```python
from build123d import *
from OCP.BRepFilletAPI import BRepFilletAPI_MakeChamfer

# Parameters (mm, degrees)
SKETCH3_W           = 20
SKETCH3_H           = 20
BOSS_EXTRUDE1_DEPTH = 2
SKETCH4_W           = 20
SKETCH4_H           = 20
SKETCH4_W_2         = 17.8
SKETCH4_H_2         = 17.8
BOSS_EXTRUDE2_DEPTH = 0.8
CHAMFER1_SIZE       = 2
BOSS_EXTRUDE3_DEPTH = 4.8
FILLET2_R           = 1
FILLET4_R           = 1
BOSS_EXTRUDE4_DEPTH = 6.1
CHAMFER2_SIZE       = 1.5
CHAMFER2_SIZE2      = 0.415986816
FILLET5_R           = 0.25
FILLET6_R           = 0.25


with BuildPart() as part:
    # Sketch3 → Boss-Extrude1 (new body)
    with BuildSketch(Plane.XY):
        Rectangle(SKETCH3_W, SKETCH3_H)
    extrude(amount=BOSS_EXTRUDE1_DEPTH)

    # Sketch4 → Boss-Extrude2 (add)
    with BuildSketch(Plane.XY.offset(2)):
        Rectangle(SKETCH4_W, SKETCH4_H)
        Rectangle(SKETCH4_W_2, SKETCH4_H_2, mode=Mode.SUBTRACT)
    extrude(amount=BOSS_EXTRUDE2_DEPTH)

    # Chamfer1
    chamfer1_edges = [part.edges().sort_by_distance(p)[0] for p in [
        (0, 10, 0),
        (10, 0, 0),
        (0, -10, 0),
        (-10, 0, 0),
    ]]
    chamfer(chamfer1_edges, length=CHAMFER1_SIZE)

    # Sketch7 → Boss-Extrude3 (add)
    with BuildSketch(Plane.XY.offset(2)):
        Polygon((-7.6, 5.05), (-7.6, -5.05), (-5.73, -5.05), (-3.861210285, -2.885), (-3.861210285, 2.885), (-5.73, 5.05), align=None)
        Polygon((-5.181210285, -2.394094045), (-5.181210285, 2.394094045), (-6.28, 3.667046113), (-6.28, -3.667046113), align=None, mode=Mode.SUBTRACT)
    boss_extrude3 = extrude(amount=BOSS_EXTRUDE3_DEPTH)

    # Mirror1: Boss-Extrude3 across plane
    add(boss_extrude3.mirror(Plane(origin=(0, 0, 0), x_dir=(0, 0, 1), z_dir=(1, 0, 0))))

    # Fillet2
    fillet2_edges = [part.edges().sort_by_distance(p)[0] for p in [
        (-6.665, 5.05, 6.8),
        (-7.6, 0, 6.8),
        (-6.665, -5.05, 6.8),
        (-4.795605142, -3.9675, 6.8),
        (-3.861210285, 0, 6.8),
        (-4.795605142, 3.9675, 6.8),
    ]]
    fillet(fillet2_edges, radius=FILLET2_R)

    # Fillet4
    fillet4_edges = [part.edges().sort_by_distance(p)[0] for p in [
        (6.665, 5.05, 6.8),
        (4.795605142, 3.9675, 6.8),
        (3.861210285, 0, 6.8),
        (4.795605142, -3.9675, 6.8),
        (6.665, -5.05, 6.8),
        (7.6, 0, 6.8),
    ]]
    fillet(fillet4_edges, radius=FILLET4_R)

    # Sketch8 → Boss-Extrude4 (add)
    with BuildSketch(Plane.XY.offset(2)):
        with BuildLine():
            Line((-0.4, 2.153160468), (-0.4, 0.4))
            Line((-0.4, 0.4), (-2.153160468, 0.4))
            ThreePointArc((-2.153160468, 0.4), (-1.548563851, 1.548563851), (-0.4, 2.153160468))
        make_face()
        with BuildLine():
            Line((0.4, 2.153160468), (0.4, 0.4))
            Line((0.4, 0.4), (2.153160468, 0.4))
            ThreePointArc((2.153160468, 0.4), (1.548563851, 1.548563851), (0.4, 2.153160468))
        make_face()
        with BuildLine():
            Line((2.153160468, -0.4), (0.4, -0.4))
            Line((0.4, -0.4), (0.4, -2.153160468))
            ThreePointArc((0.4, -2.153160468), (1.548563851, -1.548563851), (2.153160468, -0.4))
        make_face()
        with BuildLine():
            Line((-0.4, -0.4), (-2.153160468, -0.4))
            ThreePointArc((-2.153160468, -0.4), (-1.548563851, -1.548563851), (-0.4, -2.153160468))
            Line((-0.4, -2.153160468), (-0.4, -0.4))
        make_face()
    extrude(amount=BOSS_EXTRUDE4_DEPTH)

    # Chamfer2: one chamfer whose edges measure the first distance from different faces: ONE call of the kernel's chamfer builder (chamfer() names one face for all edges)
    chamfer2_edges_1 = [part.edges().sort_by_distance(p)[0] for p in [
        (1.548563851, 1.548563851, 8.1),
    ]]
    chamfer2_side_1 = [part.faces().sort_by_distance(p)[0] for p in [
        (1.548563851, 1.548563851, 5.05),
    ]]
    chamfer2_edges_2 = [part.edges().sort_by_distance(p)[0] for p in [
        (-1.548563851, 1.548563851, 8.1),
    ]]
    chamfer2_side_2 = [part.faces().sort_by_distance(p)[0] for p in [
        (-1.548563851, 1.548563851, 5.05),
    ]]
    chamfer2_edges_3 = [part.edges().sort_by_distance(p)[0] for p in [
        (1.548563851, -1.548563851, 8.1),
    ]]
    chamfer2_side_3 = [part.faces().sort_by_distance(p)[0] for p in [
        (1.548563851, -1.548563851, 5.05),
    ]]
    chamfer2_edges_4 = [part.edges().sort_by_distance(p)[0] for p in [
        (-1.548563851, -1.548563851, 8.1),
    ]]
    chamfer2_side_4 = [part.faces().sort_by_distance(p)[0] for p in [
        (-1.548563851, -1.548563851, 5.05),
    ]]
    chamfer2 = BRepFilletAPI_MakeChamfer(part.part.solid().wrapped)
    for e in chamfer2_edges_1:
        chamfer2.Add(CHAMFER2_SIZE, CHAMFER2_SIZE2, e.wrapped, chamfer2_side_1[0].wrapped)  # the first distance lies on this face
    for e in chamfer2_edges_2:
        chamfer2.Add(CHAMFER2_SIZE, CHAMFER2_SIZE2, e.wrapped, chamfer2_side_2[0].wrapped)  # the first distance lies on this face
    for e in chamfer2_edges_3:
        chamfer2.Add(CHAMFER2_SIZE, CHAMFER2_SIZE2, e.wrapped, chamfer2_side_3[0].wrapped)  # the first distance lies on this face
    for e in chamfer2_edges_4:
        chamfer2.Add(CHAMFER2_SIZE, CHAMFER2_SIZE2, e.wrapped, chamfer2_side_4[0].wrapped)  # the first distance lies on this face
    add(Compound.cast(chamfer2.Shape()), mode=Mode.REPLACE)

    # Fillet5
    # the kernel refuses this fillet: 0.25 mm, written as the material it adds along each edge
    with BuildSketch(Plane(origin=(0, 0, 2), x_dir=(0.9948253006506458, -0.10160030110857103, 0), z_dir=(-0.10160030110857103, -0.9948253006506458, 0))) as fillet5_piece_1_section:
        with BuildLine():
            CenterArc((2.19 + FILLET5_R, FILLET5_R), FILLET5_R, 180, 90)
            Line((2.19, FILLET5_R), (2.19, 0))
            Line((2.19, 0), (2.19 + FILLET5_R, 0))
        make_face()
    fillet5_piece_1 = revolve(axis=Axis((0, 0, 2), (0, 0, 1)), revolution_arc=101.662660771, mode=Mode.PRIVATE)
    fillet5_piece_1 = split(fillet5_piece_1, bisect_by=Plane(origin=(0.4, 1.598681541, 2.070877118), z_dir=(1, 0, 0)), keep=Keep.TOP, mode=Mode.PRIVATE)
    fillet5_piece_1 = split(fillet5_piece_1, bisect_by=Plane(origin=(1.598681541, 0.4, 2.070877118), z_dir=(0, 1, 0)), keep=Keep.TOP, mode=Mode.PRIVATE)
    add(fillet5_piece_1)
    with BuildSketch(Plane(origin=(0, 0, 2), x_dir=(-0.9948253006506458, -0.10160030110857048, 0), z_dir=(0.10160030110857048, -0.9948253006506458, 0))) as fillet5_piece_2_section:
        with BuildLine():
            CenterArc((2.19 + FILLET5_R, -FILLET5_R), FILLET5_R, 90, 90)
            Line((2.19, -FILLET5_R), (2.19, 0))
            Line((2.19, 0), (2.19 + FILLET5_R, 0))
        make_face()
    fillet5_piece_2 = revolve(axis=Axis((0, 0, 2), (0, 0, -1)), revolution_arc=101.662660771, mode=Mode.PRIVATE)
    fillet5_piece_2 = split(fillet5_piece_2, bisect_by=Plane(origin=(-1.598681541, 0.4, 2.070877118), z_dir=(0, 1, 0)), keep=Keep.TOP, mode=Mode.PRIVATE)
    fillet5_piece_2 = split(fillet5_piece_2, bisect_by=Plane(origin=(-0.4, 1.598681541, 2.070877118), z_dir=(-1, 0, 0)), keep=Keep.TOP, mode=Mode.PRIVATE)
    add(fillet5_piece_2)
    with BuildSketch(Plane(origin=(0, 0, 2), x_dir=(-0.1016003011085696, -0.9948253006506458, 0), z_dir=(-0.9948253006506458, 0.1016003011085696, 0))) as fillet5_piece_3_section:
        with BuildLine():
            CenterArc((2.19 + FILLET5_R, FILLET5_R), FILLET5_R, 180, 90)
            Line((2.19, FILLET5_R), (2.19, 0))
            Line((2.19, 0), (2.19 + FILLET5_R, 0))
        make_face()
    fillet5_piece_3 = revolve(axis=Axis((0, 0, 2), (0, 0, 1)), revolution_arc=101.662660771, mode=Mode.PRIVATE)
    fillet5_piece_3 = split(fillet5_piece_3, bisect_by=Plane(origin=(1.598681541, -0.4, 2.070877118), z_dir=(0, -1, 0)), keep=Keep.TOP, mode=Mode.PRIVATE)
    fillet5_piece_3 = split(fillet5_piece_3, bisect_by=Plane(origin=(0.4, -1.598681541, 2.070877118), z_dir=(1, 0, 0)), keep=Keep.TOP, mode=Mode.PRIVATE)
    add(fillet5_piece_3)
    with BuildSketch(Plane(origin=(0, 0, 2), x_dir=(-0.994825300650646, 0.10160030110856982, 0), z_dir=(0.10160030110856982, 0.994825300650646, 0))) as fillet5_piece_4_section:
        with BuildLine():
            CenterArc((2.19 + FILLET5_R, FILLET5_R), FILLET5_R, 180, 90)
            Line((2.19 + FILLET5_R, 0), (2.19, 0))
            Line((2.19, 0), (2.19, FILLET5_R))
        make_face()
    fillet5_piece_4 = revolve(axis=Axis((0, 0, 2), (0, 0, 1)), revolution_arc=101.662660771, mode=Mode.PRIVATE)
    fillet5_piece_4 = split(fillet5_piece_4, bisect_by=Plane(origin=(-0.4, -1.598681541, 2.070877118), z_dir=(-1, 0, 0)), keep=Keep.TOP, mode=Mode.PRIVATE)
    fillet5_piece_4 = split(fillet5_piece_4, bisect_by=Plane(origin=(-1.598681541, -0.4, 2.070877118), z_dir=(0, -1, 0)), keep=Keep.TOP, mode=Mode.PRIVATE)
    add(fillet5_piece_4)

    # Fillet6
    fillet6_edges = [part.edges().sort_by_distance(p)[0] for p in [
        (8, 0, 0),
        (0, 8, 0),
        (0, -8, 0),
        (-8, 0, 0),
        (-10, 10, 2.4),
        (10, 10, 2.4),
        (10, -10, 2.4),
        (-10, -10, 2.4),
    ]]
    fillet(fillet6_edges, radius=FILLET6_R)


solid = part.part
```
Can you work these out from the model? Positions are in its coordinate system, mm. A direction names the side the tool comes from. Give positions to 0.01 mm unless a question says otherwise; leave off trailing zeros. Write each loop counter-clockwise with the first axis right and the second up, starting at its lowest first coordinate (ties: lowest second). Pieces come first, ordered by that corner, then holes. Notation, with made-up numbers: (29, -17) -> (56, -17) arc R18 cw to (56, -4) -> close; hole circle Ø4 at (7.25, -20). An arc over 180 degrees is marked (long way). One line per item, written item: value.
Q1. Imagine slicing it at B-B on z = 2.5. Give the number of separate pieces and of enclosed holes in the cut face, and give its area (3 significant figures).
Results found:
separate pieces: 7
enclosed holes: 3
area: 146 mm^2
Q2. Imagine slicing it at C-C on x = 9.25. Please give me the cut outline in (y, z).
Results found:
outline: (-10, 2) -> (-9.25, 1.25) -> (9.25, 1.25) -> (10, 2) -> (10, 2.8) -> (-10, 2.8) -> close
Q3. We'd pull the mould along Y, two halves only. Please class faces 1 (the face through (-6.28, 0, 4)), 2 (the face through (1, -1, 8.1)), 3 (the face through (6.68, 4.88, 6.36)), 4 (the face through (-1.41, -1.39, 7.36)): +Y half, -Y half, draft (parallel to the pull), parting line (faces both ways), or undercut.
Results found:
face 1: undercut
face 2: draft
face 3: +Y half
face 4: -Y half
Q4. Imagine slicing it at A-A on y = 7.5. Please give me the cut outline in (x, z).
Results found:
outline: (-10, 2) -> (-8.07, 0.07) arc R0.25 ccw to (-7.9, 0) -> (7.9, 0) arc R0.25 ccw to (8.07, 0.07) -> (10, 2) -> (10, 2.8) -> (8.9, 2.8) -> (8.9, 2) -> (-8.9, 2) -> (-8.9, 2.8) -> (-10, 2.8) -> close
Q5. Which directions (+Z, -Z, +X, -X, +Y, -Y) give clear straight access to the entire face, cutting with the end or side of a thin tool? Please do faces 5 (the face through (-5.025, 3.796, 6.499)), 6 (the face through (1, 0.4, 5)), 7 (the face through (0, 0, 0)).
Results found:
face 5: +Z, +Y
face 6: +Z
face 7: -Z, +X, -X, +Y, -Y
Q6. Imagine slicing it at D-D on z = 0.5. Please give me the cut outline in (x, y).
Results found:
outline: (-8.5, -8.5) -> (8.5, -8.5) -> (8.5, 8.5) -> (-8.5, 8.5) -> close
Q7. For P1, Ø1.4, axis at x = -6, y = 1.5, coming from the +Z side; P2, Ø2.5, axis at y = 0.5, z = 3.5, coming from the +X side; P3, Ø2, axis at x = -1.5, z = 6, coming from the +Y side; P4, Ø1.5, axis at x = -0.5, y = 7, coming from the +Z side, each with a flat end and sliding along its axis, tell me the tip position at first contact or that it passes through.
Results found:
P1: stops at z = 6.8
P2: stops at x = 10
P3: stops at y = 2.13
P4: stops at z = 2
Q8. Please list where these lines run through material, in increasing order: line 1 (Y direction, x = 3.5, z = 2.75); line 2 (Z direction, x = -4.75, y = -0.25); line 3 (Z direction, x = 6, y = 6.75). Write a range as [from, to].
Results found:
line 1: y = [-10, -8.9], [8.9, 10]
line 2: z = [0, 6.79]
line 3: z = [0, 2]
